Drawing for the job (mm, zero at the part's lowest x, y, z). A direction names the side the tool comes from. Coordinates: 2 decimals unless noted, no trailing zeros. Write each loop counter-clockwise with the first axis right and the second up, starting at its lowest first coordinate (ties: lowest second). Pieces come first, ordered by that corner, then holes. Notation, with made-up numbers: M -38,-12 L 21,-12 A19 cw 21,-2 Z; hole C 6.25,-35 d2. An arc over 180 degrees is marked long. Put each result on its own line as item: value. Start each with the question number.
Q1. Pull direction Z, two halves, no side cores. Call the marked faces 4, 5 and 6: pulls with the +Z half, pulls with the -Z half, needs draft (parallel to the pull), parting line crosses it, or undercut.
Q2. Drop flat-ended pins along their axis: pin 1 (9 mm diameter, centred on y = 5, z = 7, fed in from +X); pin 2 (6.5 mm diameter, centred on y = 25, z = 7, fed in from -X); pin 3 (11 mm diameter, centred on x = 4, z = 10, fed in from +Y); pin 4 (4 mm diameter, centred on y = 5, z = 7, fed in from +X). Give the stop position or say it passes through.
Q3. Drill centre lines: line 1 along Y through (x, z) = (9.5, 7); line 2 along Z through (x, y) = (6.9, 25); line 3 along Z through (x, y) = (9.6, 25). Where is each one in solid material? Low to high.
Q4. Cut at A-A (y = 25). Write the cut outline in (x, z), then the cut area to 3 significant figures.
Q5. Cut at B-B (x = 5). Write the cut outline in (y, z).
Q6. Cut at D-D (y = 40.5). Write the cut outline in (x, z).
Q7. Which spindle directions (+Z, -Z, +X, -X, +Y, -Y) get a long thin tool onto all of the face, cutting with end or side? Do the marked faces 1, 2 and 3. Say none if no direction does.
Q8. Cut at C-C (z = 5.75). Write the cut outline in (x, y), then the cut area to 3 significant figures.
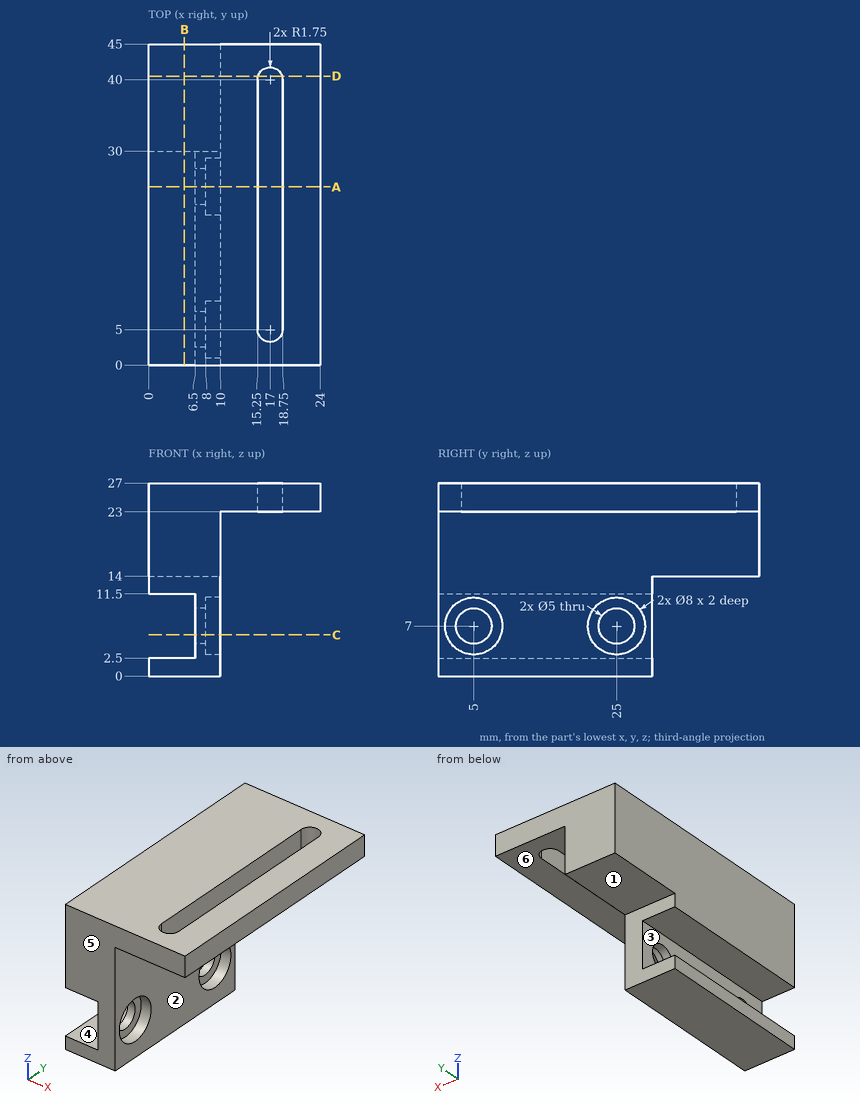
Computed values:
1. face 4: undercut
1. face 5: needs draft
1. face 6: pulls with the -Z half
2. pin 1: x = 10
2. pin 2: x = 6.5
2. pin 3: y = 45
2. pin 4: through
3. line 1: 0 to 1, 9 to 21, 29 to 30
3. line 2: 0 to 4.5, 9.5 to 27
3. line 3: 0 to 3, 11 to 27
4. outline: M 0,0 L 10,0 L 10,3 L 8,3 L 8,4.5 L 6.5,4.5 L 6.5,2.5 L 0,2.5 Z; M 0,11.5 L 6.5,11.5 L 6.5,9.5 L 8,9.5 L 8,11 L 10,11 L 10,23 L 15.25,23 L 15.25,27 L 0,27 Z; M 18.75,23 L 24,23 L 24,27 L 18.75,27 Z
4. area: 230 mm2
5. outline: M 0,0 L 30,0 L 30,2.5 L 0,2.5 Z; M 0,11.5 L 30,11.5 L 30,14 L 45,14 L 45,27 L 0,27 Z
6. outline: M 0,14 L 10,14 L 10,23 L 15.32,23 L 15.32,27 L 0,27 Z; M 18.68,23 L 24,23 L 24,27 L 18.68,27 Z
7. face 1: -Z, +X, -X, +Y
7. face 2: -Z, +X, +Y, -Y
7. face 3: -X, +Y, -Y
8. outline: M 6.5,0 L 10,0 L 10,1.2 L 8,1.2 L 8,2.83 L 6.5,2.83 Z; M 6.5,7.17 L 8,7.17 L 8,8.8 L 10,8.8 L 10,21.2 L 8,21.2 L 8,22.83 L 6.5,22.83 Z; M 6.5,27.17 L 8,27.17 L 8,28.8 L 10,28.8 L 10,30 L 6.5,30 Z
8. area: 61.6 mm2
